Geometry: final body of the model. Coordinates: model frame, mm. A direction names the side the tool comes from. Give positions to 0.01 mm unless a question says otherwise; leave off trailing zeros. Order: outer loops, then holes, each group sorted by start corner. A loop starts at its lowest first (then second) coordinate and runs counter-clockwise, first axis right, second up. Notation, with made-up numbers: (-33, -22.5) -> (-12, -22.5) arc R21 ccw to (-12, 11.5) -> close; hole circle Ø2 at (-38.75, 2.25). An arc over 180 degrees is marked (long way). One line per item, written item: value. Start each with the question number.
```python
from build123d import *

# Parameters (mm, degrees)
SKETCH1_R                = 0.3
BOSS_EXTRUDE1_DEPTH      = 2.5
BOSS_EXTRUDE2_DEPTH      = 2
BOSS_EXTRUDE2_DEPTH_BACK = 2
BOSS_EXTRUDE3_DEPTH      = 4
BOSS_EXTRUDE4_DEPTH      = 1.6
BOSS_EXTRUDE4_DEPTH_BACK = 1.6
SKETCH5_R                = 2.4
BOSS_EXTRUDE5_DEPTH      = 2.8
BOSS_EXTRUDE5_DEPTH_BACK = 2.8
SKETCH6_R                = 1.25


with BuildPart() as part:
    # Sketch1 → Boss-Extrude1 (new, symmetric)
    with BuildSketch(Plane(origin=(0, 0, 0), x_dir=(0, 0, -1), z_dir=(1, 0, 0))):
        Circle(SKETCH1_R)
    extrude(amount=BOSS_EXTRUDE1_DEPTH, both=True)

    # Sketch2 → Boss-Extrude2 (add, two sides: drawn at the far end of the back side and taken through both)
    with BuildSketch(Plane(origin=(0, 0, 0), x_dir=(0, 0, -1), z_dir=(1, 0, 0)).offset(-BOSS_EXTRUDE2_DEPTH_BACK)):
        with BuildLine():
            Line((-0.296211166, 0.047528362), (-0.296211166, 2.047528362))
            ThreePointArc((-0.296211166, 2.047528362), (-0.233869415, 2.231181239), (-0.07260959, 2.338931609))
            Line((-0.07260959, 2.338931609), (15, 6.377625177))
            Line((15, 6.377625177), (15.153330182, 5.805389146))
            Line((15.153330182, 5.805389146), (0.296211166, 1.824436104))
            Line((0.296211166, 1.824436104), (0.296211166, 0.047528362))
            Line((0.296211166, 0.047528362), (-0.296211166, 0.047528362))
        make_face()
    extrude(amount=BOSS_EXTRUDE2_DEPTH + BOSS_EXTRUDE2_DEPTH_BACK)

    # Sketch4 → Boss-Extrude3 (add)
    with BuildSketch(Plane(origin=(2, 0, 0), x_dir=(0, 0, -1), z_dir=(1, 0, 0))):
        with BuildLine():
            Line((13.22147853, 5.287751056), (17.085181835, 6.323027237))
            Line((17.085181835, 6.323027237), (16.308724699, 9.220804715))
            ThreePointArc((16.308724699, 9.220804715), (13.859234957, 10.635018278), (12.445021394, 8.185528535))
            Line((12.445021394, 8.185528535), (13.22147853, 5.287751056))
        make_face()
    extrude(amount=-BOSS_EXTRUDE3_DEPTH)

    # Sketch5 → Boss-Extrude4 (add, two sides: drawn at the far end of the back side and taken through both)
    with BuildSketch(Plane(origin=(0, 0, 0), x_dir=(0, 0, -1), z_dir=(1, 0, 0)).offset(-BOSS_EXTRUDE4_DEPTH_BACK)):
        with Locations((14.376873047, 8.703166625)):
            Circle(SKETCH5_R)
    extrude(amount=BOSS_EXTRUDE4_DEPTH + BOSS_EXTRUDE4_DEPTH_BACK)

    # Sketch6 → Boss-Extrude5 (add, two sides: drawn at the far end of the back side and taken through both)
    with BuildSketch(Plane(origin=(0, 0, 0), x_dir=(0, 0, -1), z_dir=(1, 0, 0)).offset(-BOSS_EXTRUDE5_DEPTH_BACK)):
        with Locations((14.376873047, 8.703166625)):
            Circle(SKETCH6_R)
    extrude(amount=BOSS_EXTRUDE5_DEPTH + BOSS_EXTRUDE5_DEPTH_BACK)


solid = part.part
```
1. Cut plane D-D, the plane z = -7.75. Return loops of the section in (x, y) (3 decimals), then the cut area to 3 significant figures.
2. Material intervals for L1, parallel to X at y = 5.5, z = -13.75; L2, parallel to Y at x = 0.3, z = -3.5; L3, parallel to Y at x = -0.05, z = -2.75, sorted ascending. Write a range as [from, to].
3. Pin query (flat end, axial travel): P1, Ø0.7, axis at y = 0, z = 0, coming from the +X side; P2, Ø5, axis at y = 7, z = -9, coming from the -X side; P3, Ø2, axis at x = 0, z = -2, coming from the -Y side. Return the tip coordinate at first contact, or that it passes through.
4. Cut plane C-C, the plane y = 3.5. Return loops of the section in (x, z).
5. Cut plane B-B, the plane z = -16. Return loops of the section in (x, y), then the cut area to 3 significant figures.
6. Access query for faces 1 (the cylindrical face through (2.39, 9.94, -14.21)), 2 (the cylindrical face through (-2.41, 9.94, -14.21)). Directions: +Z, -Z, +X, -X, +Y, -Y. A direction counts if a zero-diameter tool reaches every point of the face in a straight line with its end or side. Return the directions, or none.
7. Cut plane A-A, the plane x = 1.1. Return loops of the section in (y, z), then the cut area to 3 significant figures.
Answers follow:
1. outline: (-2, 3.822) -> (2, 3.822) -> (2, 4.435) -> (-2, 4.435) -> close
1. area: 2.45 mm²
2. L1: x = [-2, 2]
2. L2: y = [2.68, 3.3]
2. L3: y = [2.48, 3.1]
3. P1: stops at x = 2.5
3. P2: stops at x = -2
3. P3: stops at y = 2.01
4. outline: (-2, -6.55) -> (2, -6.55) -> (2, -4.26) -> (-2, -4.26) -> close
5. outline: (-2, 6.03) -> (2, 6.03) -> (2, 9.87) -> (1.6, 9.87) -> (1.6, 10.47) -> (-1.6, 10.47) -> (-1.6, 9.87) -> (-2, 9.87) -> close
5. area: 17.3 mm²
6. face 1: +X
6. face 2: -X
7. outline: (0.05, -0.3) -> (1.82, -0.3) -> (6.32, -17.09) -> (7.94, -16.65) arc R2.4 ccw (long way) to (6.9, -12.79) -> (5.86, -13.07) -> (2.34, 0.07) arc R0.3 ccw to (2.05, 0.3) -> (0.05, 0.3) arc R0.3 ccw (long way) to start
7. area: 31.2 mm²
